The model under review builds one solid part; all positions refer to its coordinate system, in mm. Face numbers are marked on the shaded views. A direction names the side the tool comes from. Round coordinates to 2 decimals unless told otherwise and drop trailing zeros. Write each loop counter-clockwise with the first axis right and the second up, starting at its lowest first coordinate (ties: lowest second). Pieces come first, ordered by that corner, then holes. Notation, with made-up numbers: M -36,60.5 L 23,60.5 A36 cw 23,94.5 Z; hole C 89,82 d4. An arc over 180 degrees is marked long. Write item = value, one per line. Start each with the question number.
Item 1: For pin 1 Ø1.5 at (x, y) = (2.5, 23) entering from +Z, flat-tipped, find the tip position at first contact; note if it passes through.
Item 2: Tool access review of the marked faces 1 and 2: name each direction out of +Z, -Z, +X, -X, +Y, -Y from which nothing blocks a thin tool from reaching the whole face with its end or side.
Item 3: Take a section at A-A, the plane y = 24. Give the boundary of the cut face in (x, z).
Item 4: Take a section at B-B, the plane x = 0. Give the boundary of the cut face in (y, z), plus the area to 3 significant figures.
Item 5: To check wall thickness, follow line 1 along Y through (x, z) = (0.75, 2.75); line 2 along Y through (x, z) = (-1, 2.5); line 3 along Z through (x, y) = (-1.25, 29). State the ranges of each line that lie inside material, in increasing order.
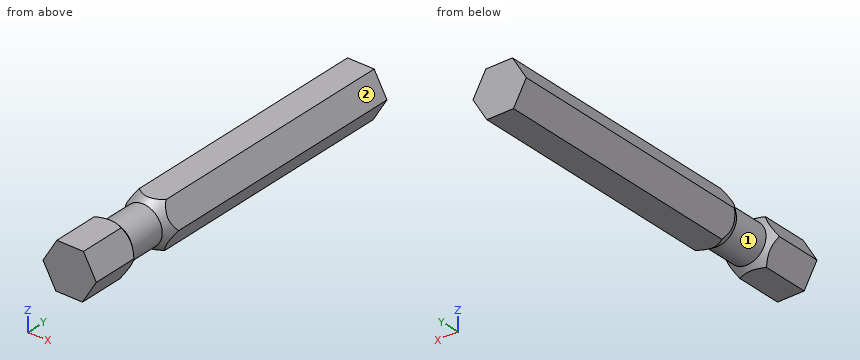
from build123d import *

# Parameters (mm, degrees)
F0_W     = 2.6
F0_H     = 5
F2_R     = 3.75
F3_DEPTH = 65


with BuildPart() as f1:
    # F0 (on Top) → F1 (revolve)
    with BuildSketch(Plane.XY):
        Polygon((-2.6, -5.1), (0, -5.1), (0, 31.73), (-3.75, 31.73), (-3.75, 17.5), (-3.75, -3.27), align=None)
        with Locations((-1.3, -7.6)):
            Rectangle(F0_W, F0_H)
        Polygon((-3.75, -11.31), (-3.75, -17.5), (0, -17.5), (0, -10.1), (-2.6, -10.1), align=None)
    revolve(axis=Axis((0, 7.115, 0), (0, -1, 0)))

    # F2 (on face) → F3 (cut)
    with BuildSketch(Plane.XZ.offset(17.5)):
        Circle(F2_R)
        Polygon((-3.578769, 0.075814), (-1.723728, 3.137212), (1.855041, 3.061398), (3.578769, -0.075814), (1.723728, -3.137212), (-1.855041, -3.061398), align=None, mode=Mode.SUBTRACT)
    extrude(amount=-F3_DEPTH, mode=Mode.SUBTRACT)


solid = f1.part
Response values:
q1.pin_1 = 3.06
q2.face_1 = none
q2.face_2 = +Z, +X, +Y, -Y
q3.outline = M -3.58,0.08 L -1.86,-3.06 L 1.72,-3.14 L 3.58,-0.08 L 1.86,3.06 L -1.72,3.14 Z
q4.outline = M -17.5,-3.1 L -10.63,-3.1 L -10.1,-2.6 L -5.1,-2.6 L -4.3,-3.1 L 31.73,-3.1 L 31.73,3.1 L -4.3,3.1 L -5.1,2.6 L -10.1,2.6 L -10.63,3.1 L -17.5,3.1 Z
q4.area = 300 mm2
q5.line_1 = -17.5 to -10.36, -4.7 to 31.73
q5.line_2 = -17.5 to -10.2, -4.95 to 31.73
q5.line_3 = -3.07 to 3.13
